Can you work these out from the model? Positions are in its coordinate system, mm. A direction names the side the tool comes from. Coordinates: 2 decimals unless noted, no trailing zeros. Order: outer loops, then holes, each group sorted by start corner. A loop starts at its lowest first (then second) coordinate and runs counter-clockwise, first axis right, second up. Notation, with made-up numbers: (29.5, 37) - (42.5, 37) arc R11 cw to (42.5, 42) - close; hole circle Ø10 at (50.5, 50.25). An arc over 180 degrees is marked (long way). Use a Markdown table: item, result. Add a question column.
(1) I want a section at B-B (x = 0). List the corners of the cut face in (y, z) for me.
(2) I want a section at C-C (z = 1.3). State how many separate pieces and enclosed holes the cut face has, and give its area (3 significant figures).
(3) For pin 1 Ø2 at (x, y) = (2.5, -7.5) entering from -Z; pin 2 Ø4 at (x, y) = (0, 0) entering from -Z, each with a flat end and sliding along its axis, tell me the tip position at first contact or that it passes through.
(4) I want a section at A-A (y = 13.5). List the corners of the cut face in (x, z) for me.
(5) On a 3-axis mill with a long thin cutter (end or side, diameter ignored), from which of +Z, -Z, +X, -X, +Y, -Y can I reach the whole of each face in a straight line? I mean faces 5 (the flat face through (12, 15, 2)), 6 (the flat face through (0, 4, 3)). Say none if no direction works.
(6) We'd pull the mould along X, two halves only. Please class faces 1 (the flat face through (-13, 15, 2)), 2 (the flat face through (25, 0, 1)), 3 (the flat face through (0, 4, 0)), 4 (the flat face through (-25, 0, 1)): pulls with the +X half, pulls with the -X half, needs draft (parallel to the pull), parting line crosses it, or undercut.
(7) If I drill on L1, parallel to Y at x = 0, z = 1.2; L2, parallel to Y at x = 15.5, z = 1.7; L3, parallel to Y at x = -13, z = 2.75, over which ranges is the centre line in solid material (lowest first)? Write a range as [from, to].
```python
from build123d import *

# Parameters (mm, degrees)
F0_W     = 50
F0_H     = 35
F1_DEPTH = 3
F2_W     = 5
F2_H     = 3
F2_R     = 3.5
F2_R_2   = 1.5
F3_DEPTH = 25


with BuildPart() as f1:
    # F0 (on Top) → F1 (new body)
    with BuildSketch(Plane.XY):
        Rectangle(F0_W, F0_H)
    extrude(amount=F1_DEPTH)

    # F2 (on face) → F3 (cut)
    with BuildSketch(Plane.XY.offset(3)):
        with Locations((-12.5, 13.5)):
            Rectangle(F2_W, F2_H)
        with Locations((12.5, 13.5)):
            Rectangle(F2_W, F2_H)
        Circle(F2_R)
        with Locations((0, 13.5)):
            Circle(F2_R_2)
        with BuildLine():
            add(Edge.make_bspline(
                [(-10, 0), (-10, 1.299038), (-17.5, 0.649519), (-25, 0), (-17.5, -0.649519), (-10, -1.299038), (-10, 0)],
                knots=[0, 0, 0, 2.094395, 2.094395, 4.18879, 4.18879, 6.283185, 6.283185, 6.283185], degree=2, weights=[1, 0.5, 1, 0.5, 1, 0.5, 1]))
        make_face()
        with BuildLine():
            add(Edge.make_bspline(
                [(10, 0), (10, -1.299038), (17.5, -0.649519), (25, 0), (17.5, 0.649519), (10, 1.299038), (10, 0)],
                knots=[0, 0, 0, 2.094395, 2.094395, 4.18879, 4.18879, 6.283185, 6.283185, 6.283185], degree=2, weights=[1, 0.5, 1, 0.5, 1, 0.5, 1]))
        make_face()
    extrude(amount=-F3_DEPTH, mode=Mode.SUBTRACT)


solid = f1.part
```
Answers follow:
| question | item | result |
|---|---|---|
| 1 | outline | (-17.5, 0) - (-3.5, 0) - (-3.5, 3) - (-17.5, 3) - close; (3.5, 0) - (12, 0) - (12, 3) - (3.5, 3) - close; (15, 0) - (17.5, 0) - (17.5, 3) - (15, 3) - close |
| 2 | separate pieces | 1 |
| 2 | enclosed holes | 6 |
| 2 | area | 1,650 mm² |
| 3 | pin 1 | stops at z = 0 |
| 3 | pin 2 | passes through |
| 4 | outline | (-25, 0) - (-15, 0) - (-15, 3) - (-25, 3) - close; (-10, 0) - (-1.5, 0) - (-1.5, 3) - (-10, 3) - close; (1.5, 0) - (10, 0) - (10, 3) - (1.5, 3) - close; (15, 0) - (25, 0) - (25, 3) - (15, 3) - close |
| 5 | face 5 | +Z, -Z |
| 5 | face 6 | +Z, +X, -X, +Y, -Y |
| 6 | face 1 | undercut |
| 6 | face 2 | pulls with the +X half |
| 6 | face 3 | needs draft |
| 6 | face 4 | pulls with the -X half |
| 7 | L1 | y = [-17.5, -3.5], [3.5, 12], [15, 17.5] |
| 7 | L2 | y = [-17.5, -0.75], [0.75, 17.5] |
| 7 | L3 | y = [-17.5, -0.69], [0.69, 12], [15, 17.5] |
